from build123d import *

# Parameters (mm, degrees)
F0_R     = 6.35
F1_DEPTH = 3.175
F2_R     = 2.06375
F3_DEPTH = 6.351
F4_R     = 2.06375
F5_DEPTH = 6.351


with BuildPart() as f1:
    # F0 (on Top) → F1 (new body, symmetric)
    with BuildSketch(Plane.XY):
        with BuildLine():
            Line((-9.525, 3.175), (-9.525, 0))
            ThreePointArc((-9.525, 0), (0, -9.525), (9.525, 0))
            Line((9.525, 0), (9.525, 3.175))
            Line((9.525, 3.175), (17.78, 3.175))
            Line((17.78, 3.175), (17.78, 9.525))
            Line((17.78, 9.525), (-17.78, 9.525))
            Line((-17.78, 9.525), (-17.78, 3.175))
            Line((-17.78, 3.175), (-9.525, 3.175))
        make_face()
        Circle(F0_R, mode=Mode.SUBTRACT)
    extrude(amount=F1_DEPTH, both=True)

    # F2 (on face) → F3 (cut, through all)
    with BuildSketch(Plane.XZ.offset(-3.175)):
        with Locations((-13.6525, 0)):
            Circle(F2_R)
    extrude(amount=-F3_DEPTH, mode=Mode.SUBTRACT)

    # F4 (on face) → F5 (cut, through all)
    with BuildSketch(Plane.XZ.offset(-3.175)):
        with Locations((13.6525, 0)):
            Circle(F4_R)
    extrude(amount=-F5_DEPTH, mode=Mode.SUBTRACT)


solid = f1.part
The listing builds one solid part. Answer for the finished solid, in the listing's coordinates (mm). A direction names the side the tool comes from. Give positions to 0.01 mm unless a question says otherwise; leave off trailing zeros. Write each loop counter-clockwise with the first axis right and the second up, starting at its lowest first coordinate (ties: lowest second). Pieces come first, ordered by that corner, then holes.
Item 1: Which of the six approach directions +Z, -Z, +X, -X, +Y, -Y give full straight-line access (tool end or side, diameter ignored) to faces 1 (the cylindrical face through (-11.746, 6.306, -0.79)), 2 (the flat face through (9.525, 2, 0)), 3 (the flat face through (-9.525, 2, 0))?
Item 2: Section C-C, the plane y = 5 is taken. Write down the section's boundary in (x, z) (1 decimal).
Item 3: Section D-D, the plane z = 2.75 is taken. Write down the section's boundary in (x, y) (3 decimals).
Item 4: Find the intervals of material crossed by line 1 along X through (y, z) = (0.25, 1.25) (3 decimals); line 2 along X through (y, z) = (4.25, 0.5); line 3 along Y through (x, z) = (-10.5, 1.5) (3 decimals), in increasing order.
Item 5: Flat-ended cylindrical pins translate along their axes: P1, Ø3.5, axis at y = 1, z = 0, coming from the +X side (3 decimals); P2, Ø1.9, axis at x = 15, z = 1.5, coming from the -Y side (3 decimals); P3, Ø2, axis at y = -7.5, z = -2, coming from the +X side. Find the tip coordinate at first contact, or state that the pin passes through.
Item 6: Section B-B, the plane x = 0 is taken. Write down the section's boundary in (y, z) (3 decimals).
Item 7: Section A-A, the plane z = 0 is taken. Write down the section's boundary in (x, y) (3 decimals), plus the area to 3 significant figures.
Item 8: Determine the mould class of faces 4 (the flat face through (-17.78, 6, 0)), 5 (the flat face through (17.78, 6, 0)), 6 (the cylindrical face through (-1.38, -6.2, -0.04)), 7 (the flat face through (-15, 3.175, 2)) for opening direction X: released by +X, released by -X, zero draft, split by the parting line, or undercut.
Completed:
1. face 1: +Y, -Y
1. face 2: +Z, -Z, +X, -Y
1. face 3: +Z, -Z, -X, -Y
2. outline: (-17.8, -3.2) - (-3.9, -3.2) - (-3.9, 3.2) - (-17.8, 3.2) - close; (3.9, -3.2) - (17.8, -3.2) - (17.8, 3.2) - (3.9, 3.2) - close; hole circle Ø4.1 at (-13.7, 0); hole circle Ø4.1 at (13.7, 0)
3. outline: (-17.78, 3.175) - (-9.525, 3.175) - (-9.525, 0) arc R9.525 ccw to (9.525, 0) - (9.525, 3.175) - (17.78, 3.175) - (17.78, 9.525) - (-17.78, 9.525) - close; hole circle Ø12.7 at (0, 0)
4. line 1: x = -9.525 to -6.345, 6.345 to 9.525
4. line 2: x = -17.78 to -15.65, -11.65 to -4.72, 4.72 to 11.65, 15.65 to 17.78
4. line 3: y = 3.175 to 9.525
5. P1: stops at x = 9.525
5. P2: stops at y = 3.175
5. P3: stops at x = 6.96
6. outline: (-9.525, -3.175) - (-6.35, -3.175) - (-6.35, 3.175) - (-9.525, 3.175) - close; (6.35, -3.175) - (9.525, -3.175) - (9.525, 3.175) - (6.35, 3.175) - close
7. outline: (-17.78, 3.175) - (-15.716, 3.175) - (-15.716, 9.525) - (-17.78, 9.525) - close; (-11.589, 3.175) - (-9.525, 3.175) - (-9.525, 0) arc R9.525 ccw to (9.525, 0) - (9.525, 3.175) - (11.589, 3.175) - (11.589, 9.525) - (-11.589, 9.525) - close; (15.716, 3.175) - (17.78, 3.175) - (17.78, 9.525) - (15.716, 9.525) - close; hole circle Ø12.7 at (0, 0)
7. area: 250 mm2
8. face 4: released by -X
8. face 5: released by +X
8. face 6: undercut
8. face 7: zero draft
